Autodesk Fusion 360 part; units mm, degrees
sketch "Sketch1" plane through (0, 0, 0) normal (0, 1, 0) x (1, 0, 0)
  circle A0 centre (0, 0) radius 68.2625 construction
  line L0 (0, 0) -> (0, -72.136) construction
  circle A1 centre (0, -72.136) radius 22.098 construction
  circle A2 centre (0, 0) radius 65.7225 construction
  circle A3 centre (0, 0) radius 66.3575
  line L1 (0, -72.136) -> (0, -101.6) construction
  line L2 (-107.95, -101.6) -> (107.95, -101.6)
  line L3 (-107.95, -101.6) -> (-62.3707, -22.6543)
  line L4 (107.95, -101.6) -> (62.3707, -22.6543)
  circle A4 centre (0, 0) radius 71.4375
  line L5 (-62.9376, -33.7962) -> (-99.1512, -96.52)
  line L6 (-99.1512, -96.52) -> (99.1512, -96.52)
  line L7 (99.1512, -96.52) -> (59.9049, -28.5434)
  line L8 (0, -96.52) -> (15.4586, -69.7449)
  line L9 (5.8659, -96.52) -> (22.4337, -67.8236)
  line L10 (22.4337, -67.8236) -> (39.0016, -96.52)
  line L11 (44.8675, -96.52) -> (27.2642, -66.0302)
  line L12 (44.8675, -96.52) -> (72.0093, -49.5089)
  line L13 (50.7334, -96.52) -> (74.9423, -54.5889)
  line L14 (27.2642, -66.0302) -> (62.4708, -66.0302)
  line L15 (37.2612, -60.9502) -> (65.4037, -60.9502)
  line L16 (0, -96.52) -> (-15.4586, -69.7449)
  line L17 (-22.4337, -67.8236) -> (-39.0016, -96.52)
  line L18 (-5.8659, -96.52) -> (-22.4337, -67.8236)
  line L19 (-44.8675, -96.52) -> (-27.2642, -66.0302)
  line L20 (-27.2642, -66.0302) -> (-62.4708, -66.0302)
  line L21 (-44.8675, -96.52) -> (-72.0093, -49.5089)
  line L22 (-50.7334, -96.52) -> (-74.9423, -54.5889)
  line L23 (-37.2612, -60.9502) -> (-65.4037, -60.9502)
  dimension "d1" = 136.525
  dimension "d2" = 72.136
  dimension "d3" = 44.196
  dimension "d7" = 131.445
  dimension "d8" = 0.635
  dimension "d9" = 101.6
  dimension "d10" = 60
  dimension "d11" = 215.9
  dimension "d14" = 5.08
  dimension "d15" = 5.08
  dimension "d16" = 5.08
  dimension "d17" = 5.08
  dimension "d30" = 30
  dimension "d31" = 5.08
  dimension "d32" = 60
  dimension "d34" = 60
  dimension "d35" = 5.08
  dimension "d36" = 5.08
  dimension "d37" = 5.08
extrude "Extrude1" add sketch "Sketch1" along normal blind 38.1 contours A3 L3 A4 L7 | A3 L4 A4 L7 | L2 L3 L4 A4 L5 L6 L7 | A4 L12 L14 L15 | L6 L7 L12 L13 | A4 L20 L21 L23 | L5 L6 L21 L22 | A4 L6 L10 L11 | A4 L6 L17 L19 | A4 L6 L8 L9 | A4 L6 L16 L18
fillet "Fillet2" radius 3.175 29 edges at (-62.9376, 19.05, 33.7962) (-99.1512, 19.05, 96.52) (99.1512, 19.05, 96.52) (62.9376, 19.05, 33.7962) (-72.0093, 19.05, 49.5089) (-65.4037, 19.05, 60.9502) (-37.2612, 19.05, 60.9502) (-74.9423, 19.05, 54.5889) (-50.7334, 19.05, 96.52) (-62.4708, 19.05, 66.0302) (-44.8675, 19.05, 96.52) (-27.2642, 19.05, 66.0302) (-39.0016, 19.05, 96.52) (-22.4337, 19.05, 67.8236) (-5.8659, 19.05, 96.52) (-15.4586, 19.05, 69.7449) (15.4586, 19.05, 69.7449) (0, 19.05, 96.52) (5.8659, 19.05, 96.52) (22.4337, 19.05, 67.8236) (39.0016, 19.05, 96.52) (27.2642, 19.05, 66.0302) (44.8675, 19.05, 96.52) (62.4708, 19.05, 66.0302) (37.2612, 19.05, 60.9502) (72.0093, 19.05, 49.5089) (65.4037, 19.05, 60.9502) (74.9423, 19.05, 54.5889) (50.7334, 19.05, 96.52)
fillet "Fillet1" radius 7.62 4 edges at (-62.3707, 19.05, 22.6543) (62.3707, 19.05, 22.6543) (107.95, 19.05, 101.6) (-107.95, 19.05, 101.6)
equation "d15 = d14"
equation "d16 = d14"
equation "d17 = d14"
equation "d31 = d14"
equation "d35 = d14"
equation "d36 = d35"
equation "d37 = d17"
Source: CAD feature listing. Evaluate the final solid. Frame: model axes, mm. A direction names the side the tool comes from. Round coordinates to 2 decimals unless told otherwise and drop trailing zeros. Write each loop counter-clockwise with the first axis right and the second up, starting at its lowest first coordinate (ties: lowest second). Pieces come first, ordered by that corner, then holes. Notation, with made-up numbers: M 82.25,86.25 L 126.25,86.25 A13 ccw 126.25,104.25 Z; hole C -28.5,46 d11. An arc over 180 degrees is marked long. Use CSV: the item, a comma, the result in double quotes. Start each with the question number.
Q1. Access query for faces 1 (the face through (-85.667, 18.783, 63.004)), 2 (the face through (-86.9, 18.8, 75.3)). Directions: +Z, -Z, +X, -X, +Y, -Y. A direction counts if a zero-diameter tool reaches every point of the face in a straight line with its end or side. Return the directions, or none.
Q2. Cut plane A-A on x = -82. Output: boundary loops of the cut face in (y, z).
Q3. Cut plane B-B on z = 86.5. Count the separate pieces of the cut face and the enclosed holes in it, plus the area to 3 significant figures.
Q4. Pull-direction query (X, two-part tool) for faces 3 (the face through (7, 0, 69)), 4 (the face through (63.031, 19.317, 36.935)), 5 (the face through (-30.64, 18.78, 82.04)), 6 (the face through (85.667, 18.783, 63.004)); classes: +X half, -X half, draft (parallel to the pull), parting line (faces both ways), or undercut.
Q5. Line query: line 1 (Z direction, x = -69.5, y = 25); line 2 (X direction, y = 18.5, z = 70); line 3 (Z direction, x = -52, y = 36). Output: solid intervals per line, ascending. Write a range as from..to.
Q6. First-contact query: P1, Ø4, axis at x = -31, z = 85.5, coming from the -Y side; P2, Ø8, axis at x = -56, y = 20.5, coming from the -Z side; P3, Ø5, axis at x = -54.5, y = 22.5, coming from the -Z side; P4, Ø6, axis at y = 27.5, z = 77, coming from the +X side. Flat tips, straight axial feed; report the tip coordinate or a pass-through.
Q7. Cut plane C-C on z = 43. Output: boundary loops of the cut face in (x, y), plus the area to 3 significant figures.
Results found:
1,face 1,"-Z, -X, +Y, -Y"
1,face 2,"+Y, -Y"
2,outline,"M 0,56.65 L 38.1,56.65 L 38.1,66.81 L 0,66.81 Z; M 0,96.52 L 38.1,96.52 L 38.1,101.6 L 0,101.6 Z"
3,separate pieces,"8"
3,enclosed holes,"0"
3,area,"1,790 mm^2"
4,face 3,"draft"
4,face 4,"undercut"
4,face 5,"undercut"
4,face 6,"+X half"
5,line 1,"35..45.16, 53.86..64.02, 96.52..101.6"
5,line 2,"-89.71..-83.84, -66.04..-60.05, -29.69..29.69, 60.05..66.04, 83.84..89.71"
5,line 3,"41.22..48.98, 60.95..66.03, 84.17..101.6"
6,P1,"y = 0"
6,P2,"z = 31.85"
6,P3,"z = 34.1"
6,P4,"x = 95.48"
7,outline,"M -74.12,0 L -68.25,0 L -68.25,38.1 L -74.12,38.1 Z; M -57.05,0 L -50.54,0 L -50.54,38.1 L -57.05,38.1 Z; M 50.54,0 L 57.05,0 L 57.05,38.1 L 50.54,38.1 Z; M 68.25,0 L 74.12,0 L 74.12,38.1 L 68.25,38.1 Z"
7,area,"943 mm^2"
